Read the model definition and answer for the solid it produces. Units are mm, in the model's axes. A direction names the side the tool comes from. Coordinates: 2 decimals unless noted, no trailing zeros. Loops run counter-clockwise (first coordinate to the right, second up) from the corner with the lowest first, then second, coordinate; pieces in that order, holes last. Notation, with made-up numbers: (86.5, 86) -> (116.5, 86) arc R21 cw to (116.5, 113) -> close; hole circle Ø11 at (39.25, 10). An arc over 180 degrees is marked (long way). Answer as a JSON object with one key per item and string values. Group by question number.
Q1. Straight lines are drawn through the part: line 1 along Y through (x, z) = (1.25, 1.75); line 2 along Y through (x, z) = (2, 3); line 3 along X through (y, z) = (-37, -0.5). For each, find the intervals that lie inside material, in ascending order. Write a range as [from, to].
Q2. For faces 1 (the flat face through (0, 1, 0)), 2 (the cylindrical face through (1.352, -25.343, -4.292)), 3 (the cylindrical face through (2.685, -5.254, -0.596)), 4 (the flat face through (0, -6, -2)), 5 (the flat face through (0, -25.95, -2)), determine the directions among +Z, -Z, +X, -X, +Y, -Y from which every point of the face is accessible in a straight line to the end or side of a thin tool.
Q3. The part is cut by section A-A on y = -36.5. Write down the section's boundary in (x, z).
Q4. Each of these flat-tipped pins is pushed along its axis until it touches: P1, Ø1.5, axis at y = -42.5, z = -0.5, coming from the +X side; P2, Ø1.5, axis at x = 2, y = -45.5, coming from the -Z side; P3, Ø4, axis at x = 1, y = -6, coming from the +Z side. Where does it stop, or does it pass through?
from build123d import *

# Parameters (mm, degrees)
SKETCH1_R            = 2.75
BOSS_EXTRUDE1_DEPTH  = 1
SKETCH2_R            = 1.5
BOSS_EXTRUDE2_DEPTH  = 1
BOSS_EXTRUDE3_START  = 1
SKETCH3_R            = 2.75
BOSS_EXTRUDE3_DEPTH  = 1
SKETCH4_R            = 1.5
BOSS_EXTRUDE4_DEPTH  = 1
BOSS_EXTRUDE5_START  = 1
SKETCH5_R            = 2.75
BOSS_EXTRUDE5_DEPTH  = 1
SKETCH6_R            = 1.5
BOSS_EXTRUDE6_DEPTH  = 1
BOSS_EXTRUDE7_START  = 1
SKETCH7_R            = 2.75
BOSS_EXTRUDE7_DEPTH  = 1
SKETCH8_R            = 1.5
BOSS_EXTRUDE8_DEPTH  = 18.75
SKETCH9_R            = 4.5
BOSS_EXTRUDE9_DEPTH  = 1.2
SKETCH10_R           = 1.5
BOSS_EXTRUDE10_DEPTH = 32.81
FILLET1_R            = 0.5
FILLET2_R            = 0.1
FILLET3_R            = 0.5
FILLET4_R            = 0.1


with BuildPart() as part:
    # Sketch1 → Boss-Extrude1 (new body)
    with BuildSketch(Plane(origin=(0, 0, 0), x_dir=(1, 0, 0), z_dir=(0, 1, 0))):
        with Locations(Location((0, 0, 0), (0, 0, 270))):
            Circle(SKETCH1_R)
    extrude(amount=BOSS_EXTRUDE1_DEPTH)

    # Sketch2 → Boss-Extrude2 (add)
    with BuildSketch(Plane.XZ):
        with Locations(Location((0, 0, 0), (0, 0, 270))):
            Circle(SKETCH2_R)
    extrude(amount=BOSS_EXTRUDE2_DEPTH)

    # Sketch3 → Boss-Extrude3 (add)
    with BuildSketch(Plane(origin=(0, -1, 0), x_dir=(-1, 0, 0), z_dir=(0, -1, 0)).offset(BOSS_EXTRUDE3_START)):
        with Locations(Location((0, 0, 0), (0, 0, 270))):
            Circle(SKETCH3_R)
    extrude(amount=-BOSS_EXTRUDE3_DEPTH)

    # Sketch4 → Boss-Extrude4 (add)
    with BuildSketch(Plane(origin=(0, -2, 0), x_dir=(-1, 0, 0), z_dir=(0, -1, 0))):
        with Locations(Location((0, 0, 0), (0, 0, 90))):
            Circle(SKETCH4_R)
    extrude(amount=BOSS_EXTRUDE4_DEPTH)

    # Sketch5 → Boss-Extrude5 (add)
    with BuildSketch(Plane(origin=(0, -3, 0), x_dir=(-1, 0, 0), z_dir=(0, -1, 0)).offset(BOSS_EXTRUDE5_START)):
        with Locations(Location((0, 0, 0), (0, 0, 270))):
            Circle(SKETCH5_R)
    extrude(amount=-BOSS_EXTRUDE5_DEPTH)

    # Sketch6 → Boss-Extrude6 (add)
    with BuildSketch(Plane.XZ.offset(4)):
        with Locations(Location((0, 0, 0), (0, 0, 270))):
            Circle(SKETCH6_R)
    extrude(amount=BOSS_EXTRUDE6_DEPTH)

    # Sketch7 → Boss-Extrude7 (add)
    with BuildSketch(Plane.XZ.offset(5).offset(BOSS_EXTRUDE7_START)):
        with Locations(Location((0, 0, 0), (0, 0, 90))):
            Circle(SKETCH7_R)
    extrude(amount=-BOSS_EXTRUDE7_DEPTH)

    # Sketch8 → Boss-Extrude8 (add)
    with BuildSketch(Plane(origin=(0, -6, 0), x_dir=(-1, 0, 0), z_dir=(0, -1, 0))):
        with Locations(Location((0, 0, 0), (0, 0, 90))):
            Circle(SKETCH8_R)
    extrude(amount=BOSS_EXTRUDE8_DEPTH)

    # Sketch9 → Boss-Extrude9 (add)
    with BuildSketch(Plane(origin=(0, -24.75, 0), x_dir=(-1, 0, 0), z_dir=(0, -1, 0))):
        with Locations(Location((0, 0, 0), (0, 0, 90))):
            Circle(SKETCH9_R)
    extrude(amount=BOSS_EXTRUDE9_DEPTH)

    # Sketch10 → Boss-Extrude10 (add)
    with BuildSketch(Plane.XZ.offset(25.95)):
        with Locations(Location((0, 0, 0), (0, 0, 270))):
            Circle(SKETCH10_R)
    extrude(amount=BOSS_EXTRUDE10_DEPTH)

    # Fillet1
    fillet1_edges = [part.edges().sort_by_distance(p)[0] for p in [
        (0, 1, -2.75),
    ]]
    fillet(fillet1_edges, radius=FILLET1_R)

    # Fillet2
    fillet2_edges = [part.edges().sort_by_distance(p)[0] for p in [
        (0, -24.75, 4.5),
        (0, -25.95, 4.5),
    ]]
    fillet(fillet2_edges, radius=FILLET2_R)

    # Fillet3
    fillet3_edges = [part.edges().sort_by_distance(p)[0] for p in [
        (0, -6, -2.75),
    ]]
    fillet(fillet3_edges, radius=FILLET3_R)

    # Fillet4
    fillet4_edges = [part.edges().sort_by_distance(p)[0] for p in [
        (0, -58.76, 1.5),
    ]]
    fillet(fillet4_edges, radius=FILLET4_R)


solid = part.part
Final values:
{
 "1": {"line 1": "y = [-25.95, -24.75], [-6, -5], [-4, -3], [-2, -1], [0, 1]", "line 2": "y = [-25.95, -24.75]", "line 3": "x = [-1.41, 1.41]"},
 "2": {"face 1": "+Z, -Z, +X, -X, +Y", "face 2": "+Y, -Y", "face 3": "+Y", "face 4": "none", "face 5": "-Y"},
 "3": {"outline": "circle Ø3 at (0, 0)"},
 "4": {"P1": "stops at x = 1.5", "P2": "stops at z = -0.83", "P3": "stops at z = 2.75"}
}
